Autodesk Inventor part; units mm, degrees
ref_plane "Work Plane1" through (0, 0, 10) normal (0, 0, 1) x (1, 0, 0)
ref_plane "YZ Plane" through (0, 0, 0) normal (1, 0, 0) x (0, 1, 0)
ref_plane "XZ Plane" through (0, 0, 0) normal (0, 1, 0) x (-1, 0, 0)
sketch "Sketch1" plane through (0, 0, 0) normal (0, 0, 1) x (1, 0, 0)
  line L0 (12.5, 0) -> (12.5, 30)
  line L1 (12.5, 30) -> (-12.5, 30)
  line L2 (-12.5, 30) -> (-12.5, 0)
  arc A0 (-12.5, 0) -> (12.5, 0) centre (0, 0) ccw
  point P0 (0, 30)
  dimension "d0" = 25
  dimension "d1" = 30
  dimension "d2" = 30
  dimension "d3" = 12.5
  dimension "d4" = 12.5
  dimension "d5" = 12.5
extrude "Extrusion1" add sketch "Sketch1" along normal blind 20
ref_plane "Work Plane1" through (0, 0, 10) normal (0, 0, 1) x (1, 0, 0)
sketch "Sketch2" plane through (0, 0, 10) normal (0, 0, 1) x (1, 0, 0)
  line L0 (6.2, 3.5796) -> (6.2, -3.5796)
  line L1 (6.2, -3.5796) -> (0, -7.1591)
  line L2 (0, -7.1591) -> (-6.2, -3.5796)
  line L3 (-6.2, -3.5796) -> (-6.2, 3.5796)
  line L4 (-6.2, 3.5796) -> (0, 7.1591)
  line L5 (0, 7.1591) -> (6.2, 3.5796)
  line L6 (12.5, 30) -> (12.5, 0)
  line L7 (-12.5, 0) -> (-12.5, 30)
  line L8 (-12.5, 30) -> (12.5, 30)
  line L9 (12.5, 30) -> (12.5, 0)
  arc A0 (-12.5, 0) -> (12.5, 0) centre (0, 0) ccw
  dimension "d9" = 12.4
extrude "Extrusion2" cut sketch "Sketch2" along normal mid plane 7 contours L0 L1 L2 L3 L4 L5
sketch "Sketch3" plane through (0, 0, 0) normal (0, 1, 0) x (-1, 0, 0)
  point P0 (0, 0)
sketch "Sketch4" plane through (0, 0, 10) normal (0, 0, 1) x (1, 0, 0)
  point P0 (0, 0)
sketch "Sketch6" plane through (0, 0, 0) normal (0, 1, 0) x (-1, 0, 0)
  line L0 (6.2, 13.5) -> (6.2, 6.5)
  line L1 (0, 13.5) -> (-6.2, 13.5)
  line L2 (6.2, 6.5) -> (-6.2, 6.5)
  line L3 (-6.2, 6.5) -> (-6.2, 13.5)
  line L4 (-6.2, 13.5) -> (6.2, 13.5)
  line L5 (6.2, 13.5) -> (6.2, 6.5)
  point P0 (0, 0)
extrude "Extrusion3" cut sketch "Sketch6" along normal blind 30
sketch "Sketch7" plane through (0, 0, 20) normal (0, 0, 1) x (1, 0, 0)
  arc A0 (-12.5, 0) -> (12.5, 0) centre (0, 0) ccw
  line L0 (12.5, 30) -> (-12.5, 30)
  line L1 (12.5, 0) -> (12.5, 30)
  point P0 (0, 4)
  dimension "d27" = 26
  dimension "d28" = 12.5
hole "Hole1" at (0, 4, 20) direction (0, 0, -1) diameter 7.5 end through all
sketch "Sketch8" plane through (-12.5, 0, 0) normal (-1, 0, 0) x (0, 0, 1)
  line L0 (7, 8) -> (13, 8)
  line L1 (13, 8) -> (13, 0)
  line L2 (13, 0) -> (7, 0)
  line L3 (7, 0) -> (7, 8)
  line L4 (0, 0) -> (0, 30)
  dimension "d21" = 6
  dimension "d22" = 8
  dimension "d23" = 7
  dimension "d24" = 0
extrude "Extrusion4" cut sketch "Sketch8" against normal blind 25
sketch "Sketch9" plane through (0, 0, 20) normal (0, 0, 1) x (1, 0, 0)
  line L0 (-10, -10) -> (10, -10)
  line L1 (10, -10) -> (10, -15)
  line L2 (10, -15) -> (-10, -15)
  line L3 (-10, -15) -> (-10, -10)
  point P0 (0, 0)
  point P1 (0, -10)
  dimension "d29" = 10
  dimension "d30" = 5
  dimension "d31" = 20
extrude "Extrusion5" cut sketch "Sketch9" against normal blind 20
equation "\"d1\" = d2"
properties part number "Acople tuerca salida"
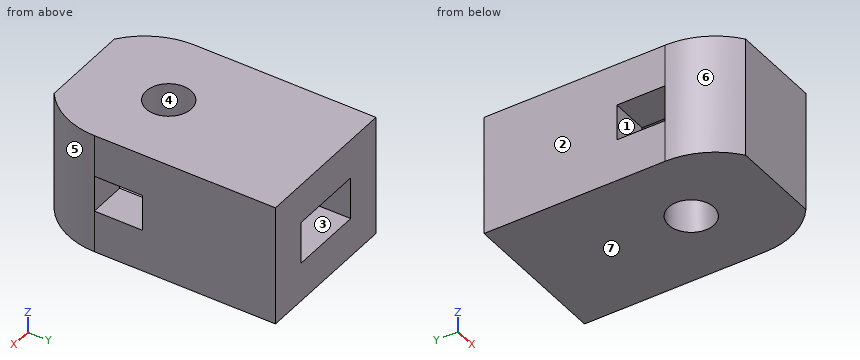
Verification items for the finished model (mm, model axes). Face numbers are marked on the shaded views. A direction names the side the tool comes from. Round coordinates to 2 decimals unless told otherwise and drop trailing zeros. Loops run counter-clockwise (first coordinate to the right, second up) from the corner with the lowest first, then second, coordinate; pieces in that order, holes last. Notation, with made-up numbers: (-33.75, -26.5) -> (11.25, -26.5) arc R22 cw to (11.25, 1.5) -> close; hole circle Ø5 at (14.5, 2.5). An arc over 180 degrees is marked (long way). Answer as a JSON object with one key per item and string values.
Q1. Section check B-B (y = 17). Record the boundary of the cut face in (x, z), then the cut area to 3 significant figures.
Data:
{"outline": "(-12.5, 0) -> (12.5, 0) -> (12.5, 20) -> (-12.5, 20) -> close; hole (-6.2, 6.5) -> (6.2, 6.5) -> (6.2, 13.5) -> (-6.2, 13.5) -> close", "area": "413 mm2"}
Q2. Scan lines: line 1 (Y direction, x = 0, z = 1.5); line 2 (Z direction, x = -5.75, y = 3); line 3 (X direction, y = 8.5, z = 8.25). Record each from-to range of solid material in increasing order. Write a range as from..to.
Data:
{"line 1": "y = -10..0.25, 7.75..30", "line 2": "z = 0..6.5, 13.5..20", "line 3": "x = -12.5..-6.2, 6.2..12.5"}
Q3. Section check A-A (z = 8.25). Record the boundary of the cut face in (x, y).
Data:
{"outline": "(-12.5, 0) arc R12.5 ccw to (-7.5, -10) -> (7.5, -10) arc R12.5 ccw to (12.5, 0) -> (6.2, 0) -> (6.2, -3.58) -> (0, -7.16) -> (-6.2, -3.58) -> (-6.2, 0) -> close; (-12.5, 8) -> (-6.2, 8) -> (-6.2, 30) -> (-12.5, 30) -> close; (6.2, 8) -> (12.5, 8) -> (12.5, 30) -> (6.2, 30) -> close"}
Q4. Section check D-D (y = 4). Record the boundary of the cut face in (x, z).
Data:
{"outline": "(-12.5, 0) -> (-3.75, 0) -> (-3.75, 6.5) -> (-6.2, 6.5) -> (-6.2, 7) -> (-12.5, 7) -> close; (-12.5, 13) -> (-6.2, 13) -> (-6.2, 13.5) -> (-3.75, 13.5) -> (-3.75, 20) -> (-12.5, 20) -> close; (3.75, 0) -> (12.5, 0) -> (12.5, 7) -> (6.2, 7) -> (6.2, 6.5) -> (3.75, 6.5) -> close; (3.75, 13.5) -> (6.2, 13.5) -> (6.2, 13) -> (12.5, 13) -> (12.5, 20) -> (3.75, 20) -> close"}
Q5. Go/stop test with flat-tipped pins: P1, Ø1.8, axis at x = 10, z = 8.5, coming from the -Y side; P2, Ø7, axis at x = 0, y = 4, coming from the +Z side. Record where each tip stops, or that it passes through.
Data:
{"P1": "stops at y = -8.57", "P2": "passes through"}
Q6. Access from +Z, -Z, +X, -X, +Y, -Y to the whole of each face (thin tool, end or side, straight path). Record for the marked faces 1, 2 and 3.
Data:
{"face 1": "+X, -X", "face 2": "+Z, -Z, -X, +Y, -Y", "face 3": "+Y"}
Q7. Section check C-C (z = 4.25). Record the boundary of the cut face in (x, y), then the cut area to 3 significant figures.
Data:
{"outline": "(-12.5, 0) arc R12.5 ccw to (-7.5, -10) -> (7.5, -10) arc R12.5 ccw to (12.5, 0) -> (12.5, 30) -> (-12.5, 30) -> close; hole circle Ø7.5 at (0, 4)", "area": "926 mm2"}
Q8. Draft check along X on the marked faces 4, 5, 6 and 7. Enter one of: pulls with the +X half, pulls with the -X half, needs draft (parallel to the pull), parting line crosses it, or undercut.
Data:
{"face 4": "undercut", "face 5": "pulls with the +X half", "face 6": "pulls with the -X half", "face 7": "needs draft"}
